```python
from build123d import *

# Parameters (mm, degrees)
F0_W     = 470
F0_H     = 470
F0_R     = 5.5
F0_R_2   = 5
F1_DEPTH = 55
F2_D     = 14
F2_DEPTH = 24
F2_TIP   = 4.2060243332
F3_R     = 100
F3_R_2   = 5
F4_DEPTH = 2
F5_R     = 12
F6_DEPTH = 30
F7_R     = 12
F8_DEPTH = 30


with BuildPart() as f1:
    # F0 (on Front) → F1 (new body)
    with BuildSketch(Plane.XZ):
        Rectangle(F0_W, F0_H)
        with Locations((-150, -150)):
            Circle(F0_R, mode=Mode.SUBTRACT)
        with Locations((150, -150)):
            Circle(F0_R, mode=Mode.SUBTRACT)
        with Locations((-150, 150)):
            Circle(F0_R, mode=Mode.SUBTRACT)
        Circle(F0_R_2, mode=Mode.SUBTRACT)
        with Locations((150, 150)):
            Circle(F0_R, mode=Mode.SUBTRACT)
    extrude(amount=F1_DEPTH)

    # F2
    with Locations(Plane(origin=(0, 0, 0), x_dir=(1, 0, 0), z_dir=(0, 1, 0))):
        with Locations((53.033008589, -53.033008589), (-53.033008589, -53.033008589), (-53.033008589, 53.033008589), (53.033008589, 53.033008589)):
            Hole(F2_D / 2, depth=F2_DEPTH)
            with Locations((0, 0, -(F2_DEPTH + F2_TIP / 2))):  # 118° drill point
                Cone(0, F2_D / 2, F2_TIP, mode=Mode.SUBTRACT)

    # F3 (on face) → F4 (cut)
    with BuildSketch(Plane.XZ):
        Circle(F3_R)
        Circle(F3_R_2, mode=Mode.SUBTRACT)
    extrude(amount=F4_DEPTH, mode=Mode.SUBTRACT)

    # F5 (on face) → F6 (cut)
    with BuildSketch(Plane.YZ.offset(235)):
        with Locations((-27.5, 0)):
            Circle(F5_R)
    extrude(amount=-F6_DEPTH, mode=Mode.SUBTRACT)

    # F7 (on face) → F8 (cut)
    with BuildSketch(Plane(origin=(-235, 0, 0), x_dir=(0, -1, 0), z_dir=(-1, 0, 0))):
        with Locations((27.5, 0)):
            Circle(F7_R)
    extrude(amount=-F8_DEPTH, mode=Mode.SUBTRACT)


solid = f1.part
```
Here's how the part is built. I have some questions about the finished solid (model axes, mm). A direction names the side the tool comes from. Round coordinates to 2 decimals unless told otherwise and drop trailing zeros. Write each loop counter-clockwise with the first axis right and the second up, starting at its lowest first coordinate (ties: lowest second). Pieces come first, ordered by that corner, then holes.
Q1. Please list where these lines run through material, in increasing order: probe 1 along Z at (x, y) = (0, -37); probe 2 along Z at (x, y) = (-150, -31); probe 3 along Z at (x, y) = (0, -1.4).
Q2. Which directions (+Z, -Z, +X, -X, +Y, -Y) give clear straight access to the entire face, cutting with the end or side of a thin tool? Please do faces 1 (the cylindrical face through (-56.796, -13.154, 47.131)), 2 (the cylindrical face through (220.21, -16.054, 3.604)), 3 (the cylindrical face through (-220.21, -38.585, -4.596)).
Q3. If we section it at A-A on z = -150: Write out the boundary of the cut face in (x, y).
Q4. If we mould it in two halves opening along Y, with no side actions, what happens to faces 4 (the cylindrical face through (53.944, -13.154, -59.973)), 5 (the flat face through (-1, -2, -21)), 6 (the flat face through (205, -28, 0))? For each: +Y half, -Y half, draft (parallel to the pull), parting line (faces both ways), or undercut.
Q5. If we section it at B-B on x = 150: Write out the boundary of the cut face in (y, z).
Q6. Will these pins go through, and if not, where does the flat tip stop? P1, Ø22.5, axis at x = 53.03, z = -53.03, coming from the +Y side; P2, Ø19, axis at y = -27.5, z = 0, coming from the +X side; P3, Ø12.5, axis at x = -53.03, z = -53.03, coming from the +Y side.
Answer below:
1. probe 1: z = -235 to -5, 5 to 235
1. probe 2: z = -235 to -155.5, -144.5 to 144.5, 155.5 to 235
1. probe 3: z = -235 to -100, 100 to 235
2. face 1: +Y
2. face 2: +X
2. face 3: -X
3. outline: (-235, -55) - (-155.5, -55) - (-155.5, 0) - (-235, 0) - close; (-144.5, -55) - (144.5, -55) - (144.5, 0) - (-144.5, 0) - close; (155.5, -55) - (235, -55) - (235, 0) - (155.5, 0) - close
4. face 4: draft
4. face 5: +Y half
4. face 6: undercut
5. outline: (-55, -235) - (0, -235) - (0, -155.5) - (-55, -155.5) - close; (-55, -144.5) - (0, -144.5) - (0, 144.5) - (-55, 144.5) - close; (-55, 155.5) - (0, 155.5) - (0, 235) - (-55, 235) - close
6. P1: stops at y = -2
6. P2: stops at x = 205
6. P3: stops at y = -24.45
